from build123d import *

# Parameters (mm, degrees)
BOSS_EXTRUDE1_DEPTH            = 350
F_3_0MM_DOWEL_HOLE1_AT_2_COUNT = 2
F_3_0MM_DOWEL_HOLE1_AT_2_PITCH = 20
F_3_0MM_DOWEL_HOLE1_AT_3_COUNT = 2
F_3_0MM_DOWEL_HOLE1_AT_3_PITCH = 23.323807579
F_3_0MM_DOWEL_HOLE1_AT_4_COUNT = 2
F_3_0MM_DOWEL_HOLE1_AT_4_PITCH = 12


with BuildPart() as part:
    # Sketch2 → Boss-Extrude1 (new body)
    with BuildSketch(Plane.XY):
        Polygon((0, 0), (0, 7), (-3, 7), (-3, -3), (43, -3), (43, 7), (40, 7), (40, 0), align=None)
    extrude(amount=BOSS_EXTRUDE1_DEPTH)

    # Sketch3 → Ø3.0mm Dowel Hole1 (revolve, cut)
    with BuildSketch(Plane(origin=(10, -3, 342), x_dir=(0, 0, -1), z_dir=(1, 0, 0))):
        Polygon((0, 0), (0, 15.901290929), (1.5, 15), (1.5, 0), align=None)
    f_3_0mm_dowel_hole1 = revolve(axis=Axis((10, -9.35, 342), (0, 1, 0)), mode=Mode.SUBTRACT)

    # Ø3.0mm Dowel Hole1 at 2: Ø3.0mm Dowel Hole1 ×2
    with Locations(*[(i * F_3_0MM_DOWEL_HOLE1_AT_2_PITCH, 0, 0) for i in range(1, F_3_0MM_DOWEL_HOLE1_AT_2_COUNT)]):
        add(f_3_0mm_dowel_hole1, mode=Mode.SUBTRACT)

    # Ø3.0mm Dowel Hole1 at 3: Ø3.0mm Dowel Hole1 ×2
    with Locations(*[Vector(0.857492926, 0, -0.514495755) * (i * F_3_0MM_DOWEL_HOLE1_AT_3_PITCH) for i in range(1, F_3_0MM_DOWEL_HOLE1_AT_3_COUNT)]):
        add(f_3_0mm_dowel_hole1, mode=Mode.SUBTRACT)

    # Ø3.0mm Dowel Hole1 at 4: Ø3.0mm Dowel Hole1 ×2
    with Locations(*[(0, 0, -i * F_3_0MM_DOWEL_HOLE1_AT_4_PITCH) for i in range(1, F_3_0MM_DOWEL_HOLE1_AT_4_COUNT)]):
        add(f_3_0mm_dowel_hole1, mode=Mode.SUBTRACT)

    # Mirror1: Ø3.0mm Dowel Hole1 across plane
    add(f_3_0mm_dowel_hole1.mirror(Plane.XY.offset(175)), mode=Mode.SUBTRACT)

    # Mirror1 copy 1 sketch → Mirror1 copy 1 (revolve, cut)
    with BuildSketch(Plane(origin=(30, -3, 8), x_dir=(0, 0, 1), z_dir=(1, 0, 0))):
        Polygon((0, 0), (0, -15.901290929), (1.5, -15), (1.5, 0), align=None)
    revolve(axis=Axis((30, -9.35, 8), (0, -1, 0)), mode=Mode.SUBTRACT)

    # Mirror1 copy 2 sketch → Mirror1 copy 2 (revolve, cut)
    with BuildSketch(Plane(origin=(30, -3, 20), x_dir=(0, 0, 1), z_dir=(1, 0, 0))):
        Polygon((0, 0), (0, -15.901290929), (1.5, -15), (1.5, 0), align=None)
    revolve(axis=Axis((30, -9.35, 20), (0, -1, 0)), mode=Mode.SUBTRACT)

    # Mirror1 copy 3 sketch → Mirror1 copy 3 (revolve, cut)
    with BuildSketch(Plane(origin=(10, -3, 20), x_dir=(0, 0, 1), z_dir=(1, 0, 0))):
        Polygon((0, 0), (0, -15.901290929), (1.5, -15), (1.5, 0), align=None)
    revolve(axis=Axis((10, -9.35, 20), (0, -1, 0)), mode=Mode.SUBTRACT)


solid = part.part
The listing builds one solid part. Answer for the finished solid, in the listing's coordinates (mm). A direction names the side the tool comes from. Coordinates: 2 decimals unless noted, no trailing zeros. Write each loop counter-clockwise with the first axis right and the second up, starting at its lowest first coordinate (ties: lowest second). Pieces come first, ordered by that corner, then holes. Notation, with made-up numbers: (-12, 78) - (-7, 78) arc R11 cw to (-7, 84) - close; hole circle Ø1 at (76.25, -21.5). An arc over 180 degrees is marked (long way). Put each result on its own line as item: value.
1. The part is cut by section A-A on z = 106. Give the vertices of the cut face in (x, y).
Answer sheet:
outline: (-3, -3) - (43, -3) - (43, 7) - (40, 7) - (40, 0) - (0, 0) - (0, 7) - (-3, 7) - close
2. A tool of negligible diameter and unlimited length cuts with its end or side. For faces 1 (the face through (20, -3, 173)), 2 (the face through (40, 4, 173)), from which of +Z, -Z, +X, -X, +Y, -Y can it reach the whole face along a straight path? Write none if from no direction.
Answer sheet:
face 1: +Z, -Z, +X, -X, -Y
face 2: +Z, -Z, +Y
3. The part is cut by section B-B on x = 18. Give the vertices of the cut face in (y, z), plus the area to 3 significant figures.
Answer sheet:
outline: (-3, 0) - (0, 0) - (0, 350) - (-3, 350) - close
area: 1,050 mm^2
4. Flat-ended cylindrical pins translate along their axes: pin 1 Ø5 at (x, z) = (30, 20) entering from +Y; pin 2 Ø1.8 at (x, z) = (10, 20) entering from -Y. Find the tip coordinate at first contact, or state that the pin passes through.
Answer sheet:
pin 1: stops at y = 0
pin 2: passes through
5. Determine the mould class of faces 3 (the face through (19.7, -0.2, 0)), 4 (the face through (-3, 2, 173)), 5 (the face through (43, 2, 173)), 6 (the face through (0, 3, 173)) for opening direction X: pulls with the +X half, pulls with the -X half, needs draft (parallel to the pull), parting line crosses it, or undercut.
Answer sheet:
face 3: needs draft
face 4: pulls with the -X half
face 5: pulls with the +X half
face 6: undercut
6. Find the intervals of material crossed by line 1 along Z through (x, y) = (10, -0.8); line 2 along X through (y, z) = (1.75, 61.5); line 3 along X through (y, z) = (-1.55, 330), in increasing order. Write a range as from..to.
Answer sheet:
line 1: z = 0..6.5, 9.5..18.5, 21.5..328.5, 331.5..340.5, 343.5..350
line 2: x = -3..0, 40..43
line 3: x = -3..8.5, 11.5..28.5, 31.5..43
